Can you work these out from the model? Positions are in its coordinate system, mm. A direction names the side the tool comes from. Round coordinates to 2 decimals unless told otherwise and drop trailing zeros. Loops run counter-clockwise (first coordinate to the right, second up) from the corner with the lowest first, then second, coordinate; pieces in that order, holes last.
```python
from build123d import *

# Parameters (mm, degrees)
F0_W     = 60
F0_H     = 40
F1_DEPTH = 15
F2_DEPTH = 5
F3_T     = -5
F4_R     = 5


with BuildPart() as f1:
    # F0 (on Top) → F1 (new body)
    with BuildSketch(Plane.XY):
        Rectangle(F0_W, F0_H)
    extrude(amount=F1_DEPTH)

    # F2 (add): a face of the model
    f2_faces = [f1.faces().sort_by_distance(p)[0] for p in [
        (0, 0, 15),
    ]]
    extrude(f2_faces, amount=F2_DEPTH)

    # F3
    f3_openings = [f1.faces().sort_by_distance(p)[0] for p in [
        (0, 0, 20),
    ]]
    offset(amount=F3_T, openings=f3_openings)

    # F4
    f4_edges = [f1.edges().sort_by_distance(p)[0] for p in [
        (-30, 20, 10),
        (-30, -20, 10),
        (30, -20, 10),
        (30, 20, 10),
        (25, 15, 12.5),
        (-25, 15, 12.5),
        (25, -15, 12.5),
        (-25, -15, 12.5),
    ]]
    fillet(f4_edges, radius=F4_R)


solid = f1.part
```
(1) Suppose I cut it at A-A (z = 18.25). Write out the boundary of the cut face in (x, y), then the cut area to 3 significant figures.
(2) For pin 1 (15 mm diameter, centred on x = -11.5, y = -0.5, fed in from +Z), with a flat end and sliding along its axis, tell me the tip position at first contact or that it passes through.
(3) If I drill on line 1 (Y direction, x = 8, z = 8.25); line 2 (X direction, y = -4, z = 9); line 3 (X direction, y = 13.5, z = 10.75), over which ranges is the centre line in solid material (lowest first)?
(4) Which directions (+Z, -Z, +X, -X, +Y, -Y) give clear straight access to the entire face, cutting with the end or side of a thin tool? Please do faces 1 (the flat face through (0, -17, 20)), 2 (the flat face through (0, 15, 12)).
(5) Suppose I cut it at B-B (x = -17). Write out the boundary of the cut face in (y, z), then the cut area to 3 significant figures.
(6) Suppose I cut it at C-C (y = -6.5). Write out the boundary of the cut face in (x, z).
(7) We'd pull the mould along Y, two halves only. Please class faces 3 (the flat face through (0, -20, 10)), 4 (the cylindrical face through (-29, 18, 10)), 5 (the flat face through (0, 0, 0)), 6 (the cylindrical face through (24, 13, 12)): released by +Y, released by -Y, zero draft, split by the parting line, or undercut.
Check result:
1. outline: (-30, -15) arc R5 ccw to (-25, -20) - (25, -20) arc R5 ccw to (30, -15) - (30, 15) arc R5 ccw to (25, 20) - (-25, 20) arc R5 ccw to (-30, 15) - close; hole (-25, -10) arc R5 ccw to (-20, -15) - (20, -15) arc R5 ccw to (25, -10) - (25, 10) arc R5 ccw to (20, 15) - (-20, 15) arc R5 ccw to (-25, 10) - close
1. area: 900 mm2
2. pin 1: stops at z = 5
3. line 1: y = -20 to -15, 15 to 20
3. line 2: x = -30 to -25, 25 to 30
3. line 3: x = -30 to -23.57, 23.57 to 30
4. face 1: +Z, +X, -X, +Y, -Y
4. face 2: +Z
5. outline: (-20, 0) - (20, 0) - (20, 20) - (15, 20) - (15, 5) - (-15, 5) - (-15, 20) - (-20, 20) - close
5. area: 350 mm2
6. outline: (-30, 0) - (30, 0) - (30, 20) - (25, 20) - (25, 5) - (-25, 5) - (-25, 20) - (-30, 20) - close
7. face 3: released by -Y
7. face 4: released by +Y
7. face 5: zero draft
7. face 6: undercut
